Geometry check sheet. Reference: the model listing, model coordinates, mm. Face numbers are marked on the shaded views. A direction names the side the tool comes from. Give positions to 0.01 mm unless a question says otherwise; leave off trailing zeros. Order: outer loops, then holes, each group sorted by start corner. A loop starts at its lowest first (then second) coordinate and runs counter-clockwise, first axis right, second up. Notation, with made-up numbers: M -39.5,63 L -28.5,63 A24 ccw -28.5,94 Z; hole C 77,56 d3. An arc over 180 degrees is marked long. Answer as CSV lines item,"result". Start each with the question number.
Q1. Set-up check for the marked faces 1 and 2: record each of +Z, -Z, +X, -X, +Y, -Y from which the full face is reachable in a straight line by a thin tool's end or side.
Q2. Section check B-B, the plane y = 56.5. Record the boundary of the cut face in (x, z).
Q3. Mould release check, pull along Y, two halves, no side actions. Record for the marked faces 3, 4 and 5: +Y half, -Y half, draft (parallel to the pull), parting line (faces both ways), or undercut.
Q4. Go/stop test with flat-tipped pins: pin 1 (1 mm diameter, centred on y = 38.5, z = 0.5, fed in from +X); pin 2 (1.4 mm diameter, centred on x = 1, z = 1, fed in from +Y); pin 3 (2 mm diameter, centred on x = -1, y = 16, fed in from +Z). Record where each tip stops, or that it passes through.
Q5. Thickness scan on line 1 (X direction, y = 26.5, z = 0.15); line 2 (Z direction, x = 0.5, y = 40.5); line 3 (X direction, y = 33.5, z = 0.95). Record the ranges inside material, lowest first.
Q6. Section check A-A, the plane y = 15. Record the boundary of the cut face in (x, z).
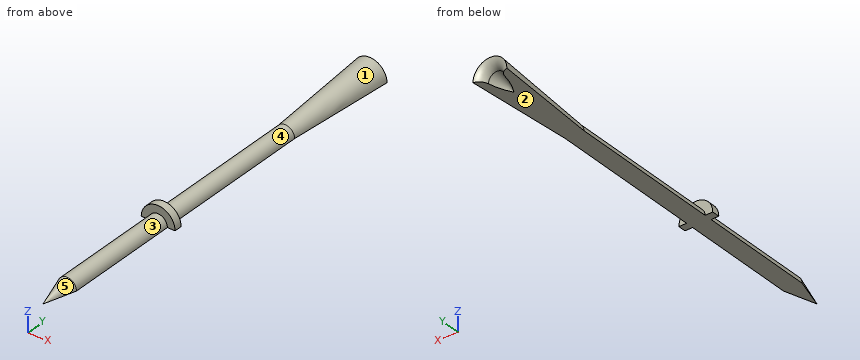
```python
from build123d import *

# Parameters (mm, degrees)
F1_ANGLE = 180


with BuildPart() as f1:
    # F0 (on Top) → F1 (revolve)
    with BuildSketch(Plane.XY):
        with BuildLine():
            Line((-1.524, 5.08), (0, 0))
            Line((0, 0), (0, 63.5))
            ThreePointArc((0, 63.5), (-0.860989, 65.238151), (-1.375962, 67.108251))
            ThreePointArc((-1.375962, 67.108251), (-1.859621, 68.048616), (-2.791716, 68.548026))
            Line((-2.791716, 68.548026), (-1.524, 50.8))
            Line((-1.524, 50.8), (-1.524, 25.4))
            Line((-1.524, 25.4), (-2.794, 25.4))
            Line((-2.794, 25.4), (-2.794, 24.13))
            Line((-2.794, 24.13), (-1.524, 24.13))
            Line((-1.524, 24.13), (-1.524, 5.08))
        make_face()
    revolve(axis=Axis((0, 31.75, 0), (0, 1, 0)), revolution_arc=F1_ANGLE)


solid = f1.part
```
Answer block:
1,face 1,"+Z"
1,face 2,"-Z, +X, -X, +Y, -Y"
2,outline,"M -1.93,0 L 1.93,0 A1.93 ccw Z"
3,face 3,"draft"
3,face 4,"undercut"
3,face 5,"-Y half"
4,pin 1,"stops at x = 1.52"
4,pin 2,"stops at y = 68.26"
4,pin 3,"stops at z = 1.52"
5,line 1,"x = -1.52 to 1.52"
5,line 2,"z = 0 to 1.44"
5,line 3,"x = -1.19 to 1.19"
6,outline,"M -1.52,0 L 1.52,0 A1.52 ccw Z"
